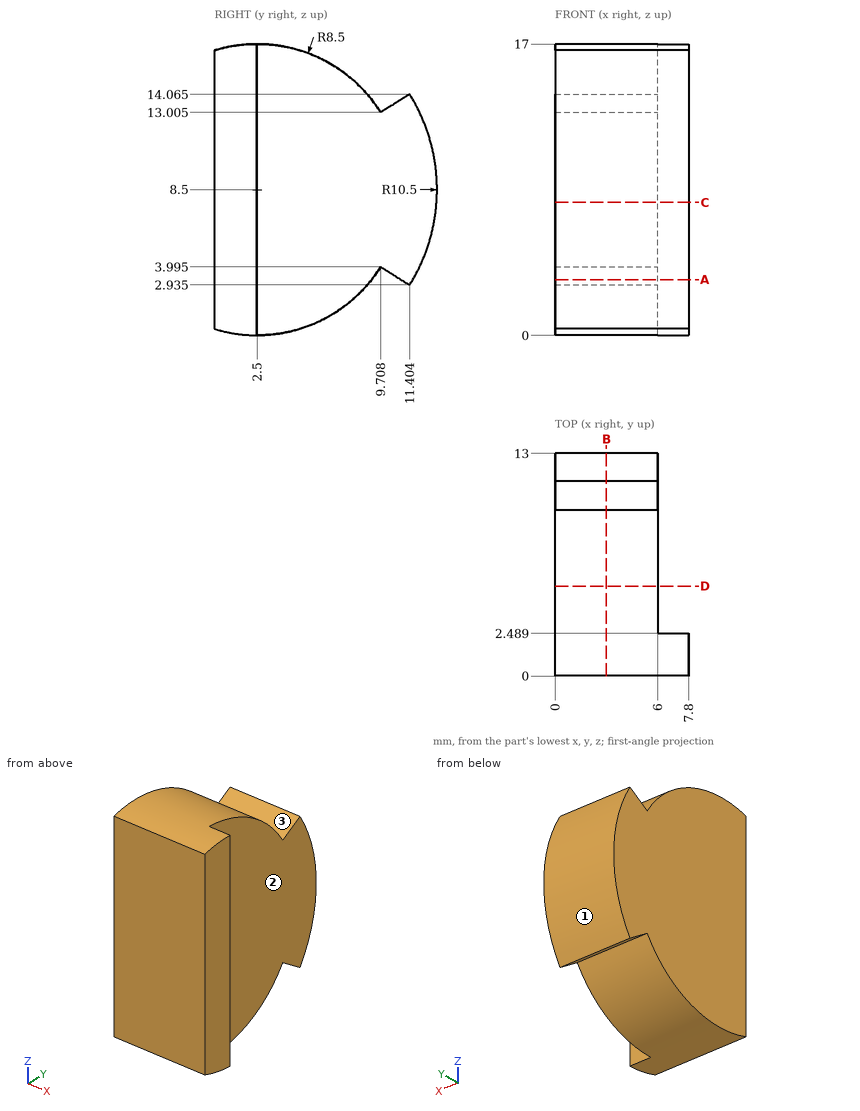
Part print with two shaded views. Sizes in mm from the minimum x, y, z corner. A direction names the side the tool comes from. Round coordinates to 2 decimals unless told otherwise and drop trailing zeros. Order: outer loops, then holes, each group sorted by start corner. A loop starts at its lowest first (then second) coordinate and runs counter-clockwise, first axis right, second up.
(1) Pin check, flat tips, straight feed: pin 1 (4 mm diameter, centred on x = 5, y = 7, fed in from +Z); pin 2 (4 mm diameter, centred on x = 2.5, y = 10, fed in from +Z); pin 3 (1.5 mm diameter, centred on x = 4.5, y = 8.5, fed in from -Z) (1 decimal); pin 4 (4 mm diameter, centred on x = 5.5, y = 3.5, fed in from -Z). Stop position of each tip, or through.
(2) Drill centre lines: line 1 (X direction, y = 4.75, z = 13.25); line 2 (Y direction, x = 6.75, z = 5.25); line 3 (Y direction, x = 2.25, z = 3.5) (1 decimal). Where is each one in solid material? Low to high.
(3) Band-saw the part on A-A (z = 3.25). List the corners of the cut face in (x, y) (1 decimal).
(4) 3-axis set-ups, long thin cutter, end or side, ignore diameter. For the marked faces 1, 2 and 3: which of +Z, -Z, +X, -X, +Y, -Y reach the whole face in a straight line?
(5) Band-saw the part on D-D (y = 5.25). List the corners of the cut face in (x, z), then the cut area to 3 significant figures.
(6) Band-saw the part on C-C (z = 7.75). List the corners of the cut face in (x, y).
(7) Band-saw the part on B-B (x = 3). List the corners of the cut face in (y, z) (1 decimal), then the cut area to 3 significant figures.
Verdict:
1. pin 1: stops at z = 16.62
1. pin 2: stops at z = 14.98
1. pin 3: stops at z = 1.8
1. pin 4: stops at z = 0
2. line 1: x = 0 to 6
2. line 2: y = 0 to 2.49
2. line 3: y = 0 to 9.4, 10.5 to 11.7
3. outline: (0, 0) - (7.8, 0) - (7.8, 2.5) - (6, 2.5) - (6, 9.2) - (0, 9.2) - close; (0, 10.9) - (6, 10.9) - (6, 11.6) - (0, 11.6) - close
4. face 1: +X, -X, +Y
4. face 2: +Z, -Z, +X, +Y
4. face 3: +Z, +X, -X
5. outline: (0, 0.46) - (6, 0.46) - (6, 16.54) - (0, 16.54) - close
5. area: 96.5 mm2
6. outline: (0, 0) - (7.8, 0) - (7.8, 2.49) - (6, 2.49) - (6, 12.97) - (0, 12.97) - close
7. outline: (0, 0.4) arc R8.5 ccw to (9.7, 4) - (11.4, 2.9) arc R10.5 ccw to (11.4, 14.1) - (9.7, 13) arc R8.5 ccw to (0, 16.6) - close
7. area: 177 mm2
